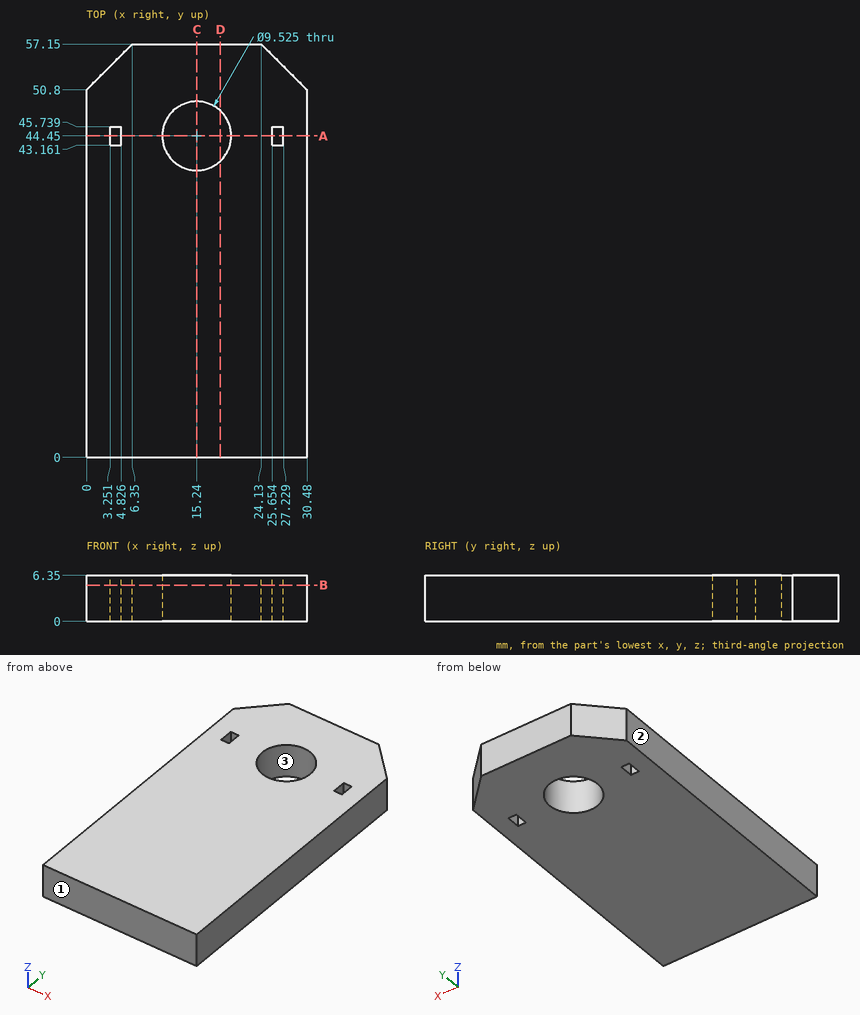
Geometry check sheet. Reference: drawing and pictorial views, mm from the part's lowest x, y, z. Coordinates: 2 decimals unless noted, no trailing zeros. Order: outer loops, then holes, each group sorted by start corner. A loop starts at its lowest first (then second) coordinate and runs counter-clockwise, first axis right, second up. Notation, with made-up numbers: (-39, -25.5) -> (5, -25.5) arc R37 cw to (5, 10.5) -> close; hole circle Ø2 at (69.5, -21.5). An arc over 180 degrees is marked (long way). Use CSV: the item, a comma, the result in double quotes. Start each with the question number.
Q1. Thickness scan on line 1 along Y through (x, z) = (15.24, 3); line 2 along Y through (x, z) = (19.5, 4.5); line 3 along X through (y, z) = (41.5, 1.25). Record the ranges inside material, lowest first.
Q2. Draft check along X on the marked faces 1, 2 and 3. Enter one of: +X half, -X half, draft (parallel to the pull), parting line (faces both ways), or undercut.
Q3. Section check C-C, the plane x = 15.24. Record the cut outline in (y, z).
Q4. Section check A-A, the plane y = 44.45. Record the cut outline in (x, z), and give its area (3 significant figures).
Q5. Section check B-B, the plane z = 5. Give the number of separate pieces and of enclosed holes in the cut face, and give its area (3 significant figures).
Q6. Depth check by flat-ended pin: P1, Ø0.8, axis at x = 3.5, z = 2, coming from the +Y side; P2, Ø5.5, axis at x = 15.24, y = 44.45, coming from the +Z side; P3, Ø0.5, axis at x = 26, z = 1.5, coming from the +Y side. Enter the tip coordinate at first touch or a pass-through.
Q7. Section check D-D, the plane x = 18.5. Record the cut outline in (y, z), and give its area (3 significant figures).
Returned:
1,line 1,"y = 0 to 39.69, 49.21 to 57.15"
1,line 2,"y = 0 to 42.32, 46.58 to 57.15"
1,line 3,"x = 0 to 11.5, 18.98 to 30.48"
2,face 1,"draft"
2,face 2,"-X half"
2,face 3,"undercut"
3,outline,"(0, 0) -> (39.69, 0) -> (39.69, 6.35) -> (0, 6.35) -> close; (49.21, 0) -> (57.15, 0) -> (57.15, 6.35) -> (49.21, 6.35) -> close"
4,outline,"(0, 0) -> (3.25, 0) -> (3.25, 6.35) -> (0, 6.35) -> close; (4.83, 0) -> (10.48, 0) -> (10.48, 6.35) -> (4.83, 6.35) -> close; (20, 0) -> (25.65, 0) -> (25.65, 6.35) -> (20, 6.35) -> close; (27.23, 0) -> (30.48, 0) -> (30.48, 6.35) -> (27.23, 6.35) -> close"
4,area,"113 mm^2"
5,separate pieces,"1"
5,enclosed holes,"3"
5,area,"1,620 mm^2"
6,P1,"stops at y = 54.7"
6,P2,"passes through"
6,P3,"stops at y = 55.53"
7,outline,"(0, 0) -> (40.98, 0) -> (40.98, 6.35) -> (0, 6.35) -> close; (47.92, 0) -> (57.15, 0) -> (57.15, 6.35) -> (47.92, 6.35) -> close"
7,area,"319 mm^2"
